```python
from build123d import *

# Parameters (mm, degrees)
SKETCH1_R           = 7
SKETCH1_R_2         = 4
BOSS_EXTRUDE1_DEPTH = 2
SKETCH2_R           = 6.2
SKETCH2_R_2         = 4.8
CUT_EXTRUDE1_DEPTH  = 0.5
CHAMFER1_SIZE       = 0.2


with BuildPart() as part:
    # Sketch1 → Boss-Extrude1 (new, symmetric)
    with BuildSketch(Plane(origin=(0, 0, 0), x_dir=(0, 0, -1), z_dir=(1, 0, 0))):
        Circle(SKETCH1_R)
        Circle(SKETCH1_R_2, mode=Mode.SUBTRACT)
    extrude(amount=BOSS_EXTRUDE1_DEPTH, both=True)

    # Sketch2 → Cut-Extrude1 (cut)
    with BuildSketch(Plane(origin=(2, 0, 0), x_dir=(0, 0, -1), z_dir=(1, 0, 0))):
        Circle(SKETCH2_R)
        Circle(SKETCH2_R_2, mode=Mode.SUBTRACT)
    cut_extrude1 = extrude(amount=-CUT_EXTRUDE1_DEPTH, mode=Mode.SUBTRACT)

    # Mirror1: Cut-Extrude1 across plane
    add(cut_extrude1.mirror(Plane(origin=(0, 0, 0), x_dir=(0, 0, 1), z_dir=(1, 0, 0))), mode=Mode.SUBTRACT)

    # Chamfer1
    chamfer1_edges = [part.edges().sort_by_distance(p)[0] for p in [
        (2, 0, 6.2),
        (2, 0, 4.8),
        (-2, 0, 4.8),
        (-2, 0, 6.2),
        (-2, 0, 7),
        (2, 0, 7),
        (-2, 0, 4),
        (2, 0, 4),
    ]]
    chamfer(chamfer1_edges, length=CHAMFER1_SIZE)


solid = part.part
```
Can you work these out from the model? Positions are in its coordinate system, mm. A direction names the side the tool comes from. Give positions to 0.01 mm unless a question says otherwise; leave off trailing zeros. Write each loop counter-clockwise with the first axis right and the second up, starting at its lowest first coordinate (ties: lowest second). Pieces come first, ordered by that corner, then holes. Notation, with made-up numbers: (88, -6) -> (134, -6) arc R15 ccw to (134, 12) -> close; hole circle Ø7 at (89.5, -11.5). An arc over 180 degrees is marked (long way). Write item = value, one per line.
(1) I'm going to push flat-ended pins straight in: P1, Ø2, axis at x = 1, z = 4, coming from the +Y side; P2, Ø7.5, axis at y = 0, z = 0, coming from the -X side; P3, Ø1, axis at x = 0, y = 3.5, coming from the -Z side; P4, Ø1.5, axis at x = 0.5, y = -5.5, coming from the +Z side. Where does each tip first touch, or does it pass through?
Worked out:
P1 = 6.32
P2 = through
P3 = -6.32
P4 = 5.14
(2) Suppose I cut it at A-A on x = -0.1. Write out the boundary of the cut face in (y, z).
Worked out:
outline = circle Ø14 at (0, 0); hole circle Ø8 at (0, 0)
(3) I need wall thicknesses on probe 1 along Y at (x, z) = (1.6, 0); probe 2 along Y at (x, z) = (0.3, 0); probe 3 along Z at (x, y) = (-1.7, -3). Which ranges of each line are inside material? Lowest first, please. Write a range as from..to.
Worked out:
probe_1 = -7..-6.2, -4.8..-4, 4..4.8, 6.2..7
probe_2 = -7..-4, 4..7
probe_3 = -6.32..-5.43, -3.75..-2.65, 2.65..3.75, 5.43..6.32
(4) For faces 1 (the face through (-0.025, -3.905, 0.867)), 2 (the face through (-1.65, -2.37, -5.73)), 3 (the face through (1.5, -4, -3)), which set-ups out of +Z, -Z, +X, -X, +Y, -Y let a thin tool reach every point of the face, with its end or its side?
Worked out:
face_1 = +X, -X
face_2 = -X
face_3 = +X
(5) Thinking about a two-plate mould opening in Y: for faces 4 (the face through (1.65, 3.24, 3.54)), 5 (the face through (0.025, -2.681, -6.466)), which applies, released by +Y, released by -Y, zero draft, split by the parting line, or undercut?
Worked out:
face_4 = undercut
face_5 = split by the parting line
